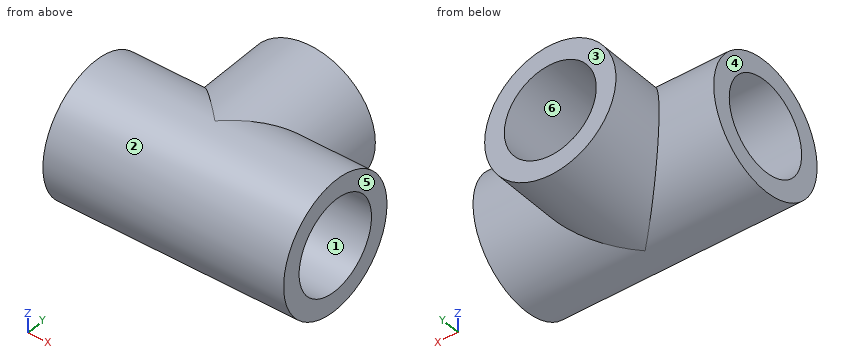
from build123d import *

# Parameters (mm, degrees)
F2_R          = 57.15
F3_DEPTH      = 104.775
F3_DEPTH_BACK = 104.775
F0_R          = 57.15
F4_DEPTH      = 104.775
F5_R          = 40.0304
F6_DEPTH      = 209.551
F1_R          = 40.0304
F7_DEPTH      = 104.776


with BuildPart() as f3:
    # F2 (on Right) → F3 (new body, two sides)
    with BuildSketch(Plane.YZ) as f3_sk:
        Circle(F2_R)
    extrude(amount=F3_DEPTH)
    extrude(f3_sk.sketch, amount=-F3_DEPTH_BACK)

    # F0 (on Front) → F4 (join)
    with BuildSketch(Plane.XZ):
        Circle(F0_R)
    extrude(amount=-F4_DEPTH)

    # F5 (on face) → F6 (cut, through all)
    with BuildSketch(Plane.YZ.offset(104.775)):
        Circle(F5_R)
    extrude(amount=-F6_DEPTH, mode=Mode.SUBTRACT)

    # F1 (on Front) → F7 (cut, through all)
    with BuildSketch(Plane.XZ):
        Circle(F1_R)
    extrude(amount=-F7_DEPTH, mode=Mode.SUBTRACT)


solid = f3.part
Read the model definition and answer for the solid it produces. Units are mm, in the model's axes. Face numbers are marked on the shaded views. A direction names the side the tool comes from. Round coordinates to 2 decimals unless told otherwise and drop trailing zeros. Order: outer loops, then holes, each group sorted by start corner. A loop starts at its lowest first (then second) coordinate and runs counter-clockwise, first axis right, second up.
1) The part is cut by section A-A on z = 0. Write down the section's boundary in (x, y) (3 decimals).
2) For the marked faces 5 and 6, determine the directions among +Z, -Z, +X, -X, +Y, -Y from which every point of the face is accessible in a straight line to the end or side of a thin tool.
3) Flat-ended cylindrical pins translate along their axes: pin 1 (10 mm diameter, centred on y = 88, z = -6.5, fed in from -X); pin 2 (1 mm diameter, centred on x = -2.5, z = 17.5, fed in from +Y); pin 3 (10 mm diameter, centred on x = 16, y = 30, fed in from -Z). Find the tip coordinate at first contact, or state that the pin passes through.
4) The mould has two halves that part along Y. Classify the marked faces 1, 2, 3 and 4: released by +Y, released by -Y, zero draft, split by the parting line, or undercut.
5) The part is cut by section B-B on y = -31.5. Write down the section's boundary in (x, z) (3 decimals).
6) Straight lines are drawn through the part: L1, parallel to Z at x = 4, y = 0; L2, parallel to Y at x = -51.5, z = -21 (3 decimals). For each, find the intervals that lie inside material, in ascending order.
7) The part is cut by section D-D on x = -44.5. Write down the section's boundary in (y, z) (3 decimals), plus the area to 3 significant figures.
8) The part is cut by section C-C on x = 0. Write down the section's boundary in (y, z) (3 decimals).
Resolved:
1. outline: (-104.775, -57.15) - (104.775, -57.15) - (104.775, -40.03) - (-104.775, -40.03) - close; (-104.775, 40.03) - (-40.03, 40.03) - (-40.03, 104.775) - (-57.15, 104.775) - (-57.15, 57.15) - (-104.775, 57.15) - close; (40.03, 40.03) - (104.775, 40.03) - (104.775, 57.15) - (57.15, 57.15) - (57.15, 104.775) - (40.03, 104.775) - close
2. face 5: +Z, -Z, +X, +Y, -Y
2. face 6: +Y
3. pin 1: stops at x = -57.13
3. pin 2: stops at y = -35.76
3. pin 3: stops at z = -56.08
4. face 1: undercut
4. face 2: split by the parting line
4. face 3: released by +Y
4. face 4: zero draft
5. outline: (-104.775, -47.685) - (104.775, -47.685) - (104.775, -24.702) - (-104.775, -24.702) - close; (-104.775, 24.702) - (104.775, 24.702) - (104.775, 47.685) - (-104.775, 47.685) - close
6. L1: z = -57.15 to -40.03, 40.03 to 57.15
6. L2: y = -53.152 to -34.08, 34.08 to 104.775
7. outline: (44.5, -35.859) - (104.775, -35.859) - (104.775, 35.859) - (44.5, 35.859) arc R57.15 ccw (long way) to start; hole circle Ø80.061 at (0, 0)
7. area: 8,930 mm2
8. outline: (0, -57.15) - (104.775, -57.15) - (104.775, -40.03) - (0, -40.03) arc R40.03 cw to (0, 40.03) - (104.775, 40.03) - (104.775, 57.15) - (0, 57.15) arc R57.15 ccw to start
